```python
from build123d import *

# Parameters (mm, degrees)
SKETCH1_W           = 6.33
SKETCH1_H           = 2.06
SKETCH1_W_2         = 0.8
SKETCH1_H_2         = 0.8
BOSS_EXTRUDE1_DEPTH = 2.5
CUT_EXTRUDE1_DEPTH  = 7.25
SKETCH3_W           = 1.42
SKETCH3_H           = 0.63
BOSS_EXTRUDE2_DEPTH = 1.21
CHAMFER1_SIZE       = 0.3


with BuildPart() as part:
    # Sketch1 → Boss-Extrude1 (new, symmetric)
    with BuildSketch(Plane(origin=(0, 0, 0), x_dir=(0, 0, -1), z_dir=(1, 0, 0))):
        Rectangle(SKETCH1_W, SKETCH1_H)
        Rectangle(SKETCH1_W_2, SKETCH1_H_2, mode=Mode.SUBTRACT)
        with Locations((-1.72, 0)):
            Rectangle(SKETCH1_W_2, SKETCH1_H_2, mode=Mode.SUBTRACT)
        with Locations((1.72, 0)):
            Rectangle(SKETCH1_W_2, SKETCH1_H_2, mode=Mode.SUBTRACT)
    extrude(amount=BOSS_EXTRUDE1_DEPTH, both=True)

    # Sketch2 → Cut-Extrude1 (cut)
    with BuildSketch(Plane.XY.offset(3.165)):
        Polygon((-1.2, 2.722191774), (0.15, 2.722191774), (0.15, 0.43), (-1.2, 0.93), align=None)
    extrude(amount=-CUT_EXTRUDE1_DEPTH, mode=Mode.SUBTRACT)

    # Sketch3 → Boss-Extrude2 (add)
    with BuildSketch(Plane(origin=(-1.2, 0, 0), x_dir=(0, 0, -1), z_dir=(1, 0, 0))):
        with Locations((-2.055, 0.715)):
            Rectangle(SKETCH3_W, SKETCH3_H)
        with Locations((0, 0.715)):
            Rectangle(SKETCH3_W, SKETCH3_H)
        with Locations((2.055, 0.715)):
            Rectangle(SKETCH3_W, SKETCH3_H)
    extrude(amount=BOSS_EXTRUDE2_DEPTH)

    # Chamfer1
    chamfer1_edges = [part.edges().sort_by_distance(p)[0] for p in [
        (-2.5, 0, -0.4),
        (-2.5, 0.4, 0),
        (-2.5, 0, 0.4),
        (-2.5, -0.4, 0),
        (2.5, 0, -0.4),
        (2.5, 0.4, 0),
        (2.5, 0, 0.4),
        (2.5, -0.4, 0),
        (-2.5, 0, 1.32),
        (-2.5, 0.4, 1.72),
        (-2.5, 0, 2.12),
        (-2.5, -0.4, 1.72),
        (2.5, 0, 1.32),
        (2.5, 0.4, 1.72),
        (2.5, 0, 2.12),
        (2.5, -0.4, 1.72),
        (-2.5, 0, -2.12),
        (-2.5, 0.4, -1.72),
        (-2.5, 0, -1.32),
        (-2.5, -0.4, -1.72),
        (2.5, 0, -2.12),
        (2.5, 0.4, -1.72),
        (2.5, 0, -1.32),
        (2.5, -0.4, -1.72),
    ]]
    chamfer(chamfer1_edges, length=CHAMFER1_SIZE)


solid = part.part
```
Check sheet for the modelled part. Datum: model origin and axes. Units: mm. A direction names the side the tool comes from. Coordinates: 2 decimals unless noted, no trailing zeros. Loops run counter-clockwise (first coordinate to the right, second up) from the corner with the lowest first, then second, coordinate; pieces in that order, holes last.
1) Release check for a two-part mould opening along Z. For faces 3 (the face through (0, -0.4, 1.7)), 4 (the face through (0, 0, -3.165)), 5 (the face through (-1, 1.03, 0)) record: released by +Z, released by -Z, zero draft, split by the parting line, or undercut.
2) Access from +Z, -Z, +X, -X, +Y, -Y to the whole of each face (thin tool, end or side, straight path). Record for faces 1 (the face through (1, 1.03, 0)), 2 (the face through (0, -0.4, -1.7)).
3) Sectioned sample at B-B (z = 0). Record the boundary of the cut face in (x, y), and give its area (3 significant figures).
4) Sectioned sample at D-D (z = -2.25). Record the boundary of the cut face in (x, y).
5) Material ranges on probe 1 along Z at (x, y) = (0.8, -0.2) (3 decimals); probe 2 along Y at (x, z) = (-1.7, 0); probe 3 along X at (y, z) = (0.35, -0.5), recorded low to high.
6) Sectioned sample at A-A (y = 0.05). Record the boundary of the cut face in (x, z) (3 decimals), and give its area (3 significant figures).
7) Sectioned sample at C-C (x = 0.35). Record the boundary of the cut face in (y, z) (3 decimals).
Check sheet entries:
1. face 3: undercut
1. face 4: released by -Z
1. face 5: zero draft
2. face 1: +Z, -Z, +X, -X, +Y
2. face 2: +X, -X
3. outline: (-2.5, -1.03) - (2.5, -1.03) - (2.5, -0.7) - (2.2, -0.4) - (-2.2, -0.4) - (-2.5, -0.7) - close; (-2.5, 0.7) - (-2.2, 0.4) - (2.2, 0.4) - (2.5, 0.7) - (2.5, 1.03) - (0.15, 1.03) - (0.15, 0.43) - (0.01, 0.48) - (0.01, 1.03) - (-2.5, 1.03) - close
3. area: 6.04 mm2
4. outline: (-2.5, -1.03) - (2.5, -1.03) - (2.5, -0.7) - (2.33, -0.53) - (2.33, 0.53) - (2.5, 0.7) - (2.5, 1.03) - (0.15, 1.03) - (0.15, 0.43) - (0.01, 0.48) - (0.01, 1.03) - (-2.5, 1.03) - (-2.5, 0.7) - (-2.33, 0.53) - (-2.33, -0.53) - (-2.5, -0.7) - close
5. probe 1: z = -3.165 to -2.12, -1.32 to -0.4, 0.4 to 1.32, 2.12 to 3.165
5. probe 2: y = -1.03 to -0.4, 0.4 to 1.03
5. probe 3: x = -2.3 to 2.3
6. outline: (-2.5, -3.165) - (2.5, -3.165) - (2.5, -2.42) - (2.2, -2.12) - (-2.2, -2.12) - (-2.5, -2.42) - close; (-2.5, -1.02) - (-2.2, -1.32) - (2.2, -1.32) - (2.5, -1.02) - (2.5, -0.7) - (2.2, -0.4) - (-2.2, -0.4) - (-2.5, -0.7) - close; (-2.5, 0.7) - (-2.2, 0.4) - (2.2, 0.4) - (2.5, 0.7) - (2.5, 1.02) - (2.2, 1.32) - (-2.2, 1.32) - (-2.5, 1.02) - close; (-2.5, 2.42) - (-2.2, 2.12) - (2.2, 2.12) - (2.5, 2.42) - (2.5, 3.165) - (-2.5, 3.165) - close
6. area: 19.1 mm2
7. outline: (-1.03, -3.165) - (1.03, -3.165) - (1.03, 3.165) - (-1.03, 3.165) - close; hole (-0.4, -2.12) - (0.4, -2.12) - (0.4, -1.32) - (-0.4, -1.32) - close; hole (-0.4, -0.4) - (0.4, -0.4) - (0.4, 0.4) - (-0.4, 0.4) - close; hole (-0.4, 1.32) - (0.4, 1.32) - (0.4, 2.12) - (-0.4, 2.12) - close
